Build history of the part. All positions in model axes, mm. A direction names the side the tool comes from. Give positions to 0.01 mm unless a question says otherwise; leave off trailing zeros. Write each loop counter-clockwise with the first axis right and the second up, starting at its lowest first coordinate (ties: lowest second). Pieces come first, ordered by that corner, then holes. Notation, with made-up numbers: (14, 15.25) -> (43, 15.25) arc R23 cw to (43, 36.25) -> close; hole circle Ø4 at (63.5, 13.25). An arc over 180 degrees is marked (long way). Write item = value, one per line. Start each with the question number.
Q1. Drop flat-ended pins along their axis: P1, Ø5, axis at y = -2, z = -46, coming from the +X side; P2, Ø8, axis at x = 8, z = 21, coming from the +Y side; P3, Ø10, axis at y = 31, z = -31, coming from the +X side. Give the stop position or say it passes through.
Q2. Saw through at C-C, the plane z = 37. List the corners of the cut face in (x, y).
Q3. Wall check: line 1 (Y direction, x = 0, z = -46); line 2 (X direction, y = 0, z = -48); line 3 (Z direction, x = -27, y = 17.5). Give the ranges that are in metal, low to high.
Q4. Tool access for faces 1 (the face through (5, 0, -46)), 2 (the face through (-3.233, -1.341, -39.815)), 3 (the face through (6.466, -2.681, 43.182)): list every direction of +Z, -Z, +X, -X, +Y, -Y with a clear straight run to the whole face (end or side of a thin tool).
Q5. Mould opens along Y. For faces 4 (the face through (16, 44, -21)), 5 (the face through (-81.075, -25.532, 0.042)), 6 (the face through (0, 0, -17)) say: pulls with the +Y half, pulls with the -Y half, needs draft (parallel to the pull), parting line crosses it, or undercut.
Q6. Saw through at B-B, the plane z = -42. List the corners of the cut face in (x, y).
from build123d import *

# Parameters (mm, degrees)
SKETCH_1_R           = 85
EXTRUDE_1_DEPTH      = 21
SKETCH_2_R           = 47
EXTRUDE_2_DEPTH      = 30
CHAMFER_1_SIZE       = 10
SKETCH_3_R           = 7
EXTRUDE_3_DEPTH      = 32
SKETCH_5_OUTSIDE_W   = 223.484
SKETCH_5_OUTSIDE_H   = 223.484
SKETCH_5_OUTSIDE_W_2 = 10
SKETCH_5_OUTSIDE_H_2 = 14
CUT_EXTRUDE_1_DEPTH  = 28
CHAMFER_3_SIZE       = 1
SKETCH_7_R           = 3.5
CUT_EXTRUDE_2_DEPTH  = 45
SKETCH_8_R           = 7
CUT_EXTRUDE_4_DEPTH  = 5
FILLET_1_R           = 18
EXTRUDE_START        = 26
SKETCH_10_R          = 7
EXTRUDE_4_DEPTH      = 26


with BuildPart() as part:
    # 草图1 → 凸台-拉伸1 (new, symmetric)
    with BuildSketch(Plane.XY):
        with Locations(Location((0, 0, 0), (0, 0, 180))):
            Circle(SKETCH_1_R)
    extrude(amount=EXTRUDE_1_DEPTH, both=True)

    # 草图2 → 凸台-拉伸2 (add, symmetric)
    with BuildSketch(Plane.XY):
        Circle(SKETCH_2_R)
    extrude(amount=EXTRUDE_2_DEPTH, both=True)

    # 倒角1
    # the kernel refuses this chamfer: 10 mm, written as the material it takes off along each edge
    with BuildSketch(Plane(origin=(0, 0, -30), x_dir=(1, 0, 0), z_dir=(0, -1, 0))) as chamfer_1_piece_1_section:
        Polygon((47, CHAMFER_1_SIZE), (47 - CHAMFER_1_SIZE, 0), (47, 0), align=None)
    chamfer_1_piece_1 = revolve(axis=Axis((0, 0, -30), (0, 0, 1)), mode=Mode.PRIVATE)
    chamfer_1_piece_1 = split(chamfer_1_piece_1, bisect_by=Plane(origin=(-41.532222796, 0, -21), z_dir=(0, 0, -1)), keep=Keep.TOP, mode=Mode.PRIVATE)
    add(chamfer_1_piece_1, mode=Mode.SUBTRACT)
    with BuildSketch(Plane(origin=(0, 0, 30), x_dir=(1, 0, 0), z_dir=(0, -1, 0))) as chamfer_1_piece_2_section:
        Polygon((47, -CHAMFER_1_SIZE), (47 - CHAMFER_1_SIZE, 0), (47, 0), align=None)
    chamfer_1_piece_2 = revolve(axis=Axis((0, 0, 30), (0, 0, 1)), mode=Mode.PRIVATE)
    chamfer_1_piece_2 = split(chamfer_1_piece_2, bisect_by=Plane(origin=(-41.532222796, 0, 21), z_dir=(0, 0, 1)), keep=Keep.TOP, mode=Mode.PRIVATE)
    add(chamfer_1_piece_2, mode=Mode.SUBTRACT)

    # 草图3 → 凸台-拉伸3 (add)
    with BuildSketch(Plane(origin=(0, 0, -30), x_dir=(-1, 0, 0), z_dir=(0, 0, -1))):
        with Locations(Location((0, 0, 0), (0, 0, 180))):
            Circle(SKETCH_3_R)
    extrude(amount=EXTRUDE_3_DEPTH)

    # 草图5 outside → 切除-拉伸1 (cut)
    with BuildSketch(Plane(origin=(0, 0, -62), x_dir=(-1, 0, 0), z_dir=(0, 0, -1))):
        Rectangle(SKETCH_5_OUTSIDE_W, SKETCH_5_OUTSIDE_H)
        Rectangle(SKETCH_5_OUTSIDE_W_2, SKETCH_5_OUTSIDE_H_2, mode=Mode.SUBTRACT)
    extrude(amount=-CUT_EXTRUDE_1_DEPTH, mode=Mode.SUBTRACT)

    # 倒角3
    # the kernel refuses this chamfer: 1 mm, written as the material it takes off along each edge
    with BuildSketch(Plane(origin=(0, 0, -62), x_dir=(-0.9180065533872216, 0.39656521271805273, 0), z_dir=(-0.39656521271805273, -0.9180065533872216, 0))) as chamfer_3_piece_1:
        Polygon((7, -CHAMFER_3_SIZE), (7 - CHAMFER_3_SIZE, 0), (7, 0), align=None)
    revolve(axis=Axis((0, 0, -62), (0, 0, -1)), revolution_arc=66.636371816, mode=Mode.SUBTRACT)
    with BuildSketch(Plane(origin=(0, 0, -62), x_dir=(0.9180065533873013, -0.3965652127178682, 0), z_dir=(0.3965652127178682, 0.9180065533873013, 0))) as chamfer_3_piece_2:
        Polygon((7, -CHAMFER_3_SIZE), (7 - CHAMFER_3_SIZE, 0), (7, 0), align=None)
    revolve(axis=Axis((0, 0, -62), (0, 0, -1)), revolution_arc=66.636371927, mode=Mode.SUBTRACT)
    with BuildSketch(Plane(origin=(0, 0, -62), x_dir=(-1.935452947399645e-09, -1.0, 0), z_dir=(1.0, -1.935452947399645e-09, 0))) as chamfer_3_piece_3:
        Polygon((7, -CHAMFER_3_SIZE), (7 - CHAMFER_3_SIZE, 0), (7, 0), align=None)
    revolve(axis=Axis((0, 0, -62), (0, 0, -1)), revolution_arc=66.636371706, mode=Mode.SUBTRACT)
    with BuildSketch(Plane(origin=(0, 0, -62), x_dir=(0, 1, 0), z_dir=(-1, 0, 0))) as chamfer_3_piece_4:
        Polygon((7, -CHAMFER_3_SIZE), (7 - CHAMFER_3_SIZE, 0), (7, 0), align=None)
    revolve(axis=Axis((0, 0, -62), (0, 0, -1)), revolution_arc=66.636371816, mode=Mode.SUBTRACT)

    # 草图7 → 切除-拉伸2 (cut)
    with BuildSketch(Plane(origin=(0, 0, -62), x_dir=(-1, 0, 0), z_dir=(0, 0, -1))):
        Circle(SKETCH_7_R)
    extrude(amount=-CUT_EXTRUDE_2_DEPTH, mode=Mode.SUBTRACT)

    # 草图8 → 切除-拉伸4 (cut)
    with BuildSketch(Plane(origin=(5, 0, 0), x_dir=(0, 0, -1), z_dir=(1, 0, 0))):
        with Locations((62, 0)):
            Circle(SKETCH_8_R)
    extrude(amount=-CUT_EXTRUDE_4_DEPTH, mode=Mode.SUBTRACT)

    # 圆角1
    fillet_1_edges = [part.edges().sort_by_distance(p)[0] for p in [
        (85, 0, -21),
        (85, 0, 21),
    ]]
    fillet(fillet_1_edges, radius=FILLET_1_R)

    # 草图10 → 凸台-拉伸4 (add)
    with BuildSketch(Plane.XY.offset(30).offset(EXTRUDE_START)):
        Circle(SKETCH_10_R)
    extrude(amount=-EXTRUDE_4_DEPTH)


solid = part.part
Report:
q1.P1 = 5
q1.P2 = 77.92
q1.P3 = 28.57
q2.outline = circle Ø14 at (0, 0)
q3.line_1 = -7 to -3.5, 3.5 to 7
q3.line_2 = -5 to -3.5, 3.5 to 5
q3.line_3 = -30 to 30
q4.face_1 = -Z, +X, +Y, -Y
q4.face_2 = -Z
q4.face_3 = +Z
q5.face_4 = needs draft
q5.face_5 = parting line crosses it
q5.face_6 = undercut
q6.outline = (-5, -4.9) arc R7 ccw to (5, -4.9) -> (5, 4.9) arc R7 ccw to (-5, 4.9) -> close; hole circle Ø7 at (0, 0)
